Geometry: final body of the model. Coordinates: model frame, mm. A direction names the side the tool comes from. Give positions to 0.01 mm unless a question says otherwise; leave off trailing zeros. Write each loop counter-clockwise with the first axis right and the second up, starting at its lowest first coordinate (ties: lowest second). Pieces come first, ordered by that corner, then holes. Notation, with made-up numbers: M 81,67.25 L 86,67.25 A25 cw 86,101.25 Z; hole C 26,72 d5. An arc over 180 degrees is marked long. Use a Markdown table: item, result. Add a question column.
1) Set-up query: faces 4 (the flat face through (256, 38, -0.605)), 5 (the flat face through (-119.735, 301, 349)), 6 (the flat face through (257, 6.35, 129)). Return all of +Z, -Z, +X, -X, +Y, -Y with unobstructed straight access to the full face (end or side cutting, diameter ignored); none if empty.
2) Pin query (flat end, axial travel): pin 1 (5 mm diameter, centred on x = 414, y = 4.5, fed in from -Z); pin 2 (5 mm diameter, centred on x = 228, z = 525, fed in from -Y). Return the tip coordinate at first contact, or that it passes through.
3) Draft query along Z for faces 1 (the flat face through (257, 6.35, 659)), 2 (the flat face through (256, 301, 786.795)), 3 (the flat face through (256, 0, 216)). Return one class per face: +Z half, -Z half, draft (parallel to the pull), parting line (faces both ways), or undercut.
4) Section A-A on x = 203. Return the cut outline in (y, z), then the cut area to 3 significant figures.
5) Line query: line 1 (Z direction, x = 281.5, y = 31); line 2 (Y direction, x = 290.5, z = 174.5); line 3 (Y direction, x = 170, z = -14.5). Output: solid intervals per line, ascending.
```python
from build123d import *

# Parameters (mm, degrees)
F0_W     = 762
F0_H     = 101.6
F0_H_2   = 258.16306
F0_W_2   = 635
F0_H_3   = 131.16306
F0_H_4   = 3.175
F0_H_5   = 65.47612
F0_H_6   = 65.68694
F1_DEPTH = 609.6
F2_DEPTH = 6.35
F3_DEPTH = 76.2


# Not quite as in the source:
# - a feature names something its author has since deleted; it is built from what else it names


with BuildPart() as f1:
    # F0 (on Front) → F1 (new body)
    with BuildSketch(Plane.XZ):
        with Locations((261.2652602196, -51.4053403184)):
            Rectangle(F0_W, F0_H)
        with Locations((261.2652602196, 128.4761896816)):
            Rectangle(F0_W, F0_H_2)
        with Locations((261.2652602196, 128.4761896816)):
            Rectangle(F0_W_2, F0_H_3, mode=Mode.SUBTRACT)
        with Locations((261.2652602196, 259.1452196816)):
            Rectangle(F0_W, F0_H_4)
        with Locations((261.2652602196, 262.3202196816)):
            Rectangle(F0_W, F0_H_4)
        Polygon((-119.7347397804, 263.9077196816), (642.2652602196, 263.9077196816), (642.2652602196, 393.0946596816), (578.7652602196, 393.0946596816), (578.7652602196, 327.4077196816), (-56.2347397804, 327.4077196816), (-56.2347397804, 393.0946596816), (-119.7347397804, 393.0946596816), align=None)
        Polygon((578.7652602196, 393.0946596816), (642.2652602196, 393.0946596816), (642.2652602196, 522.2815996816), (-119.7347397804, 522.2815996816), (-119.7347397804, 393.0946596816), (-56.2347397804, 393.0946596816), (-56.2347397804, 458.5707796816), (578.7652602196, 458.5707796816), align=None)
        with Locations((261.2652602196, 523.8690996816)):
            Rectangle(F0_W, F0_H_4)
        with Locations((261.2652602196, 527.0440996816)):
            Rectangle(F0_W, F0_H_4)
        with Locations((261.2652602196, 657.7131296816)):
            Rectangle(F0_W, F0_H_2)
        with Locations((261.2652602196, 657.9239496816)):
            Rectangle(F0_W_2, F0_H_3, mode=Mode.SUBTRACT)
        with Locations((261.2652602196, 657.9239496816)):
            Rectangle(F0_W_2, F0_H_3)
        with Locations((261.2652602196, 425.8327196816)):
            Rectangle(F0_W_2, F0_H_5)
        with Locations((261.2652602196, 360.2511896816)):
            Rectangle(F0_W_2, F0_H_6)
        with Locations((261.2652602196, 128.4761896816)):
            Rectangle(F0_W_2, F0_H_3)
    extrude(amount=-F1_DEPTH)

    # F0 (on Front) → F2 (cut)
    with BuildSketch(Plane.XZ):
        with Locations((261.2652602196, 657.9239496816)):
            Rectangle(F0_W_2, F0_H_3)
        with Locations((261.2652602196, 425.8327196816)):
            Rectangle(F0_W_2, F0_H_5)
        with Locations((261.2652602196, 360.2511896816)):
            Rectangle(F0_W_2, F0_H_6)
        with Locations((261.2652602196, 128.4761896816)):
            Rectangle(F0_W_2, F0_H_3)
        with Locations((261.2652602196, 262.3202196816)):
            Rectangle(F0_W, F0_H_4)
        with Locations((261.2652602196, 259.1452196816)):
            Rectangle(F0_W, F0_H_4)
        with Locations((261.2652602196, 527.0440996816)):
            Rectangle(F0_W, F0_H_4)
        with Locations((261.2652602196, 523.8690996816)):
            Rectangle(F0_W, F0_H_4)
    extrude(amount=-F2_DEPTH, mode=Mode.SUBTRACT)

    # F0 (on Front) → F3 (cut)
    with BuildSketch(Plane.XZ):
        with Locations((261.2652602196, -51.4053403184)):
            Rectangle(F0_W, F0_H)
    extrude(amount=-F3_DEPTH, mode=Mode.SUBTRACT)


solid = f1.part
```
Found:
| question | item | result |
|---|---|---|
| 1 | face 4 | -Z, +X, -X, -Y |
| 1 | face 5 | +Z, -Z, -X, +Y, -Y |
| 1 | face 6 | -Y |
| 2 | pin 1 | z = -0.61 |
| 2 | pin 2 | y = 6.35 |
| 3 | face 1 | undercut |
| 3 | face 2 | +Z half |
| 3 | face 3 | draft |
| 4 | outline | M 0,-0.61 L 76.2,-0.61 L 76.2,-102.21 L 609.6,-102.21 L 609.6,786.79 L 0,786.79 L 0,723.51 L 6.35,723.51 L 6.35,592.34 L 0,592.34 L 0,528.63 L 6.35,528.63 L 6.35,522.28 L 0,522.28 L 0,458.57 L 6.35,458.57 L 6.35,327.41 L 0,327.41 L 0,263.91 L 6.35,263.91 L 6.35,257.56 L 0,257.56 L 0,194.06 L 6.35,194.06 L 6.35,62.89 L 0,62.89 Z |
| 4 | area | 532,000 mm² |
| 5 | line 1 | -0.61 to 786.79 |
| 5 | line 2 | 6.35 to 609.6 |
| 5 | line 3 | 76.2 to 609.6 |
